from build123d import *

# Parameters (mm, degrees)
EXTRUDE_2_DEPTH     = 20
SKETCH_4_W          = 4.1
SKETCH_4_H          = 5
CUT_EXTRUDE_1_DEPTH = 23
SKETCH_5_W          = 4.959838708
SKETCH_5_H          = 5
CUT_EXTRUDE_2_DEPTH = 23
SKETCH_6_R          = 1.6
CUT_EXTRUDE_3_DEPTH = 23


with BuildPart() as part:
    # 草图1 → 凸台-拉伸2 (new body)
    with BuildSketch(Plane(origin=(0, 0, 0), x_dir=(1, 0, 0), z_dir=(0, 1, 0))):
        with BuildLine():
            ThreePointArc((2.520080646, 0.75), (3.550862325, -0.34582971), (5, -0.75))
            Line((5, -0.75), (5, 0.75))
            Line((5, 0.75), (2.520080646, 0.75))
        make_face()
        with BuildLine():
            Line((5, 0.75), (5, -0.75))
            ThreePointArc((5, -0.75), (6.979898987, 0.070101013), (7.8, 2.05))
            ThreePointArc((7.8, 2.05), (4.330587642, 4.768802511), (2.520080646, 0.75))
            Line((2.520080646, 0.75), (5, 0.75))
        make_face()
        with BuildLine():
            ThreePointArc((2.520080646, 0.75), (3.550862325, -0.34582971), (5, -0.75))
            Line((5, -0.75), (5, 0.75))
            Line((5, 0.75), (2.520080646, 0.75))
        make_face()
        with BuildLine():
            Line((5, 0.75), (5, -0.75))
            ThreePointArc((5, -0.75), (6.979898987, 0.070101013), (7.8, 2.05))
            ThreePointArc((7.8, 2.05), (4.330587642, 4.768802511), (2.520080646, 0.75))
            Line((2.520080646, 0.75), (5, 0.75))
        make_face()
        with BuildLine():
            Line((-5, 0.75), (-5, -0.75))
            Line((-5, -0.75), (5, -0.75))
            ThreePointArc((5, -0.75), (3.550862325, -0.34582971), (2.520080646, 0.75))
            Line((2.520080646, 0.75), (-5, 0.75))
        make_face()
    extrude(amount=EXTRUDE_2_DEPTH)

    # 草图4 → 切除-拉伸1 (cut)
    with BuildSketch(Plane.ZY.offset(5)):
        with Locations((-2.8, 17.5)):
            Rectangle(SKETCH_4_W, SKETCH_4_H)
        with Locations((-2.8, 7.5)):
            Rectangle(SKETCH_4_W, SKETCH_4_H)
    extrude(amount=-CUT_EXTRUDE_1_DEPTH, mode=Mode.SUBTRACT)

    # 草图5 → 切除-拉伸2 (cut)
    with BuildSketch(Plane(origin=(0, 0, -0.75), x_dir=(-1, 0, 0), z_dir=(0, 0, -1))):
        with Locations((-5, 7.5)):
            Rectangle(SKETCH_5_W, SKETCH_5_H)
        with Locations((-5, 17.5)):
            Rectangle(SKETCH_5_W, SKETCH_5_H)
    extrude(amount=-CUT_EXTRUDE_2_DEPTH, mode=Mode.SUBTRACT)

    # 草图6 → 切除-拉伸3 (cut)
    with BuildSketch(Plane(origin=(0, 0, -0.75), x_dir=(-1, 0, 0), z_dir=(0, 0, -1))):
        with Locations((1.239959677, 16)):
            Circle(SKETCH_6_R)
        with Locations((1.239959677, 4)):
            Circle(SKETCH_6_R)
    extrude(amount=-CUT_EXTRUDE_3_DEPTH, mode=Mode.SUBTRACT)


solid = part.part
Source: CAD feature listing. Evaluate the final solid. Frame: model axes, mm. A direction names the side the tool comes from. Coordinates: 2 decimals unless noted, no trailing zeros. Loops run counter-clockwise (first coordinate to the right, second up) from the corner with the lowest first, then second, coordinate; pieces in that order, holes last. Notation, with made-up numbers: (54, -10.5) - (90, -10.5) arc R20 cw to (90, 14.5) - close; hole circle Ø11 at (-35, -38.5). An arc over 180 degrees is marked (long way). Return JSON: item names as keys, results as strings.
Q1. Contact query for flat-ended pins moving along their axis: P1, Ø6, axis at x = 0, y = 11, coming from the -Z side; P2, Ø3, axis at x = 6.5, z = -3, coming from the +Y side; P3, Ø1.6, axis at y = 7.5, z = 0.5, coming from the +X side; P4, Ø2.5, axis at x = -1.24, y = 16, coming from the -Z side. Output: stop coordinate, or through.
Results:
{"P1": "z = -4.01", "P2": "y = 15", "P3": "x = 2.52", "P4": "through"}
Q2. Mould query, pull axis X, two halves, no side actions, for faces 4 (the flat face through (-5, 10, 0)), 5 (the cylindrical face through (-1.98, 2.58, -0.01)), 6 (the flat face through (5, 10, -2)), 7 (the cylindrical face through (-1.032, 17.586, -0.01)). Classes: released by +X, released by -X, zero draft, split by the parting line, or undercut.
Results:
{"face 4": "released by -X", "face 5": "undercut", "face 6": "zero draft", "face 7": "undercut"}
Q3. Section C-C, the plane z = -3. Return loops of the section in (x, y).
Results:
{"outline": "(2.37, 0) - (7.63, 0) - (7.63, 5) - (2.37, 5) - close; (2.37, 10) - (7.63, 10) - (7.63, 15) - (2.37, 15) - close"}
Q4. Section A-A, the plane y = 16. Return loops of the section in (x, z), plus the area to 3 significant figures.
Results:
{"outline": "(-5, -0.75) - (-2.84, -0.75) - (-2.84, 0.75) - (-5, 0.75) - close; (0.36, -0.75) - (2.52, -0.75) - (2.52, 0.75) - (0.36, 0.75) - close", "area": "6.48 mm2"}
Q5. Access query for faces 1 (the flat face through (2.52, 17, 0)), 2 (the flat face through (0, 10, 0.75)), 3 (the flat face through (2.52, 7, 0)). Directions: +Z, -Z, +X, -X, +Y, -Y. A direction counts if a zero-diameter tool reaches every point of the face in a straight line with its end or side. Return the directions, or none.
Results:
{"face 1": "+Z, -Z, +X, +Y", "face 2": "+Z, +X, -X, +Y, -Y", "face 3": "+Z, -Z, +X"}
Q6. Material intervals for line 1 along Y through (x, z) = (3, -2.7); line 2 along X through (y, z) = (7.25, -0.1); line 3 along Z through (x, y) = (0.25, 6.75), sorted ascending.
Results:
{"line 1": "0 to 5, 10 to 15", "line 2": "-5 to 2.52", "line 3": "-0.75 to 0.75"}
Q7. Section D-D, the plane z = -0.25. Return loops of the section in (x, y).
Results:
{"outline": "(-5, 0) - (7.14, 0) - (7.14, 5) - (2.52, 5) - (2.52, 10) - (7.14, 10) - (7.14, 15) - (2.52, 15) - (2.52, 20) - (-5, 20) - close; hole circle Ø3.2 at (-1.24, 4); hole circle Ø3.2 at (-1.24, 16)"}
Q8. Section B-B, the plane x = -0.75. Return loops of the section in (y, z).
Results:
{"outline": "(0, -0.75) - (2.48, -0.75) - (2.48, 0.75) - (0, 0.75) - close; (5.52, -0.75) - (14.48, -0.75) - (14.48, 0.75) - (5.52, 0.75) - close; (17.52, -0.75) - (20, -0.75) - (20, 0.75) - (17.52, 0.75) - close"}
